Drawing for the job (mm, zero at the part's lowest x, y, z). Give positions to 0.01 mm unless a question says otherwise; leave off trailing zeros. Order: outer loops, then holes, each group sorted by start corner. A loop starts at its lowest first (then second) coordinate and runs counter-clockwise, first axis right, second up. Notation, with made-up numbers: (56.25, 15) - (109.25, 15) arc R22 ccw to (109.25, 45) - close; hole circle Ø1 at (88.25, 14). An arc over 180 degrees is marked (long way). One line per item, written item: value.
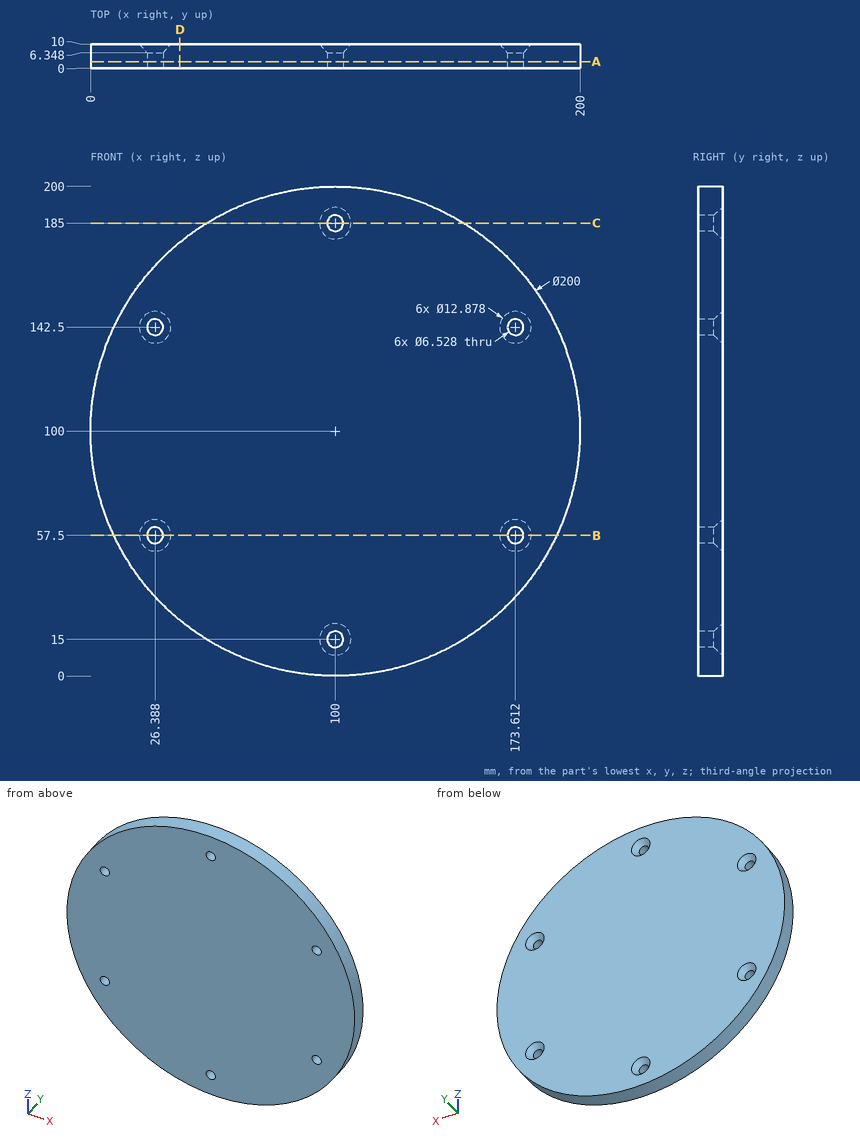
(1) Slice it at A-A, the plane y = 2.75. Give the cut face in (x, z), and give its area (3 significant figures).
Completed:
outline: circle Ø200 at (100, 100); hole circle Ø6.53 at (26.39, 57.5); hole circle Ø6.53 at (26.39, 142.5); hole circle Ø6.53 at (100, 15); hole circle Ø6.53 at (100, 185); hole circle Ø6.53 at (173.61, 57.5); hole circle Ø6.53 at (173.61, 142.5)
area: 31,200 mm²
(2) Pin check, flat tips, straight feed: P1, Ø7.5, axis at x = 26.39, z = 142.5, coming from the +Y side; P2, Ø1.5, axis at x = 68.5, y = 7, coming from the +Z side (1 decimal); P3, Ø3, axis at x = 42.5, y = 4.5, coming from the -Z side. Stop position of each tip, or through.
Completed:
P1: y = 6.91
P2: z = 195.2
P3: z = 17.15
(3) Slice it at B-B, the plane z = 57.5. Give the cut face in (x, y).
Completed:
outline: (9.48, 0) - (23.12, 0) - (23.12, 6.35) - (19.95, 10) - (9.48, 10) - close; (29.65, 0) - (170.35, 0) - (170.35, 6.35) - (167.17, 10) - (32.83, 10) - (29.65, 6.35) - close; (176.88, 0) - (190.52, 0) - (190.52, 10) - (180.05, 10) - (176.88, 6.35) - close
(4) Drill centre lines: line 1 (Z direction, x = 100.5, y = 1.5) (1 decimal); line 2 (X direction, y = 3, z = 57.5) (1 decimal); line 3 (X direction, y = 4, z = 15) (1 decimal). Where is each one in solid material? Low to high.
Completed:
line 1: 0 to 11.8, 18.2 to 181.8, 188.2 to 200
line 2: 9.5 to 23.1, 29.7 to 170.3, 176.9 to 190.5
line 3: 47.3 to 96.7, 103.3 to 152.7
(5) Slice it at C-C, the plane z = 185. Give the cut face in (x, y).
Completed:
outline: (47.32, 0) - (96.74, 0) - (96.74, 6.35) - (93.56, 10) - (47.32, 10) - close; (103.26, 0) - (152.68, 0) - (152.68, 10) - (106.44, 10) - (103.26, 6.35) - close
(6) Slice it at D-D, the plane x = 36.5. Give the cut face in (y, z), and give its area (4 significant figures).
Completed:
outline: (0, 22.75) - (10, 22.75) - (10, 177.25) - (0, 177.25) - close
area: 1,545 mm²
